```python
from build123d import *

# Parameters (mm, degrees)
PAD_DEPTH       = 30
POCKET_DEPTH    = 5
FILLET_R        = 14.5
FILLET001_R     = 14.5
FILLET002_R     = 12
SKETCH002_W     = 50.00223
SKETCH002_H     = 7.321129
PAD001_DEPTH    = 25
SKETCH003_R     = 4.8367523299
POCKET001_DEPTH = 10


with BuildPart() as part:
    # Sketch → Pad (new body)
    with BuildSketch(Plane.XY):
        Polygon((-26.0423896161, -2.4126467386), (-26.0423896161, 2.4126467386), (26.0423896161, 2.4126467386), (70.4083759206, -14.101078257), (69.0323338509, -17.9166155839), (26.0423896161, -2.4126467386), align=None)
    extrude(amount=PAD_DEPTH)

    # Sketch001 (on Face3 of Pad) → Pocket (cut)
    with BuildSketch(Plane(origin=(3.9577363848, 10.6329055553, 0), x_dir=(-0.9371842108, 0.3488348534, 0), z_dir=(0.3488348534, 0.9371842108, 0))):
        with BuildLine():
            ThreePointArc((-57.051074, 19.2972875988), (-61.3483615988, 15), (-57.051074, 10.7027124012))
            Line((-57.051074, 10.7027124012), (-38.086853, 10.7027124012))
            ThreePointArc((-38.086853, 10.7027124012), (-33.7895654012, 15), (-38.086853, 19.2972875988))
            Line((-38.086853, 19.2972875988), (-57.051074, 19.2972875988))
        make_face()
    extrude(amount=-POCKET_DEPTH, mode=Mode.SUBTRACT)

    # Fillet
    fillet_edges = [part.edges().sort_by_distance(p)[0] for p in [
        (69.720355, -16.008847, 30),
    ]]
    fillet(fillet_edges, radius=FILLET_R)

    # Fillet001
    fillet001_edges = [part.edges().sort_by_distance(p)[0] for p in [
        (69.720355, -16.008847, 0),
    ]]
    fillet(fillet001_edges, radius=FILLET001_R)

    # Fillet002
    fillet002_edges = [part.edges().sort_by_distance(p)[0] for p in [
        (26.04239, 2.412647, 15),
    ]]
    fillet(fillet002_edges, radius=FILLET002_R)

    # Sketch002 (on Face12 of Fillet002) → Pad001 (join)
    with BuildSketch(Plane(origin=(0, 2.4126467386, 0), x_dir=(-1, 0, 0), z_dir=(0, 1, 0))):
        with Locations((1.1177492, 26.194347)):
            Rectangle(SKETCH002_W, SKETCH002_H)
    extrude(amount=PAD001_DEPTH)

    # Sketch003 (on Face17 of Pad001) → Pocket001 (cut)
    with BuildSketch(Plane.XY.offset(29.8549115)):
        with Locations((10.379424, 18.289026)):
            Circle(SKETCH003_R)
        with BuildLine():
            Line((-30.0109383074, -0.5137681689), (-30.0109383074, 32.26572))
            Line((31.0117, 32.26572), (-30.0109383074, 32.26572))
            Line((32.17643, 11.966219), (31.0117, 32.26572))
            Line((23.690575, 12.964556), (32.17643, 11.966219))
            ThreePointArc((23.690575, 12.964556), (14.0178466447, 26.3039488372), (-2.2418022126, 23.6346991039))
            Line((-2.2418022126, 23.6346991039), (-30.0109383074, -0.5137681689))
        make_face()
    extrude(amount=-POCKET001_DEPTH, mode=Mode.SUBTRACT)


solid = part.part
```
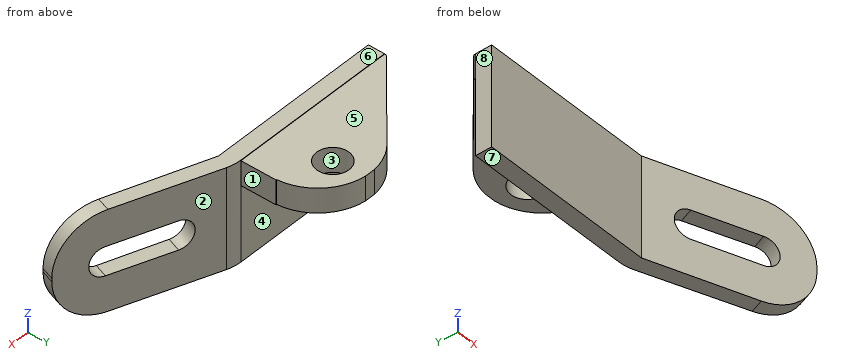
Here's how the part is built. I have some questions about the finished solid (model axes, mm). Face numbers are marked on the shaded views. A direction names the side the tool comes from. Coordinates: 2 decimals unless noted, no trailing zeros. Loops run counter-clockwise (first coordinate to the right, second up) from the corner with the lowest first, then second, coordinate; pieces in that order, holes last. Notation, with made-up numbers: (24.5, 4) - (66.5, 4) arc R25 cw to (66.5, 16) - close; hole circle Ø11 at (62, -25). An arc over 180 degrees is marked (long way). Return JSON: item names as keys, results as strings. Group by question number.
Item 1: If we section it at C-C on y = 17: Write out the boundary of the cut face in (x, z), and give its area (3 significant figures).
Item 2: If we section it at A-A on z = 24: Write out the boundary of the cut face in (x, y), and give its area (3 significant figures).
Item 3: Will these pins go through, and if not, where does the flat tip stop? P1, Ø15, axis at x = -7, z = 14, coming from the -Y side; P2, Ø2, axis at y = -3, z = 6, coming from the -X side; P3, Ø5, axis at x = 15.5, z = 21, coming from the +Y side.
Item 4: If we section it at B-B on x = 50.5: Write out the boundary of the cut face in (y, z).
Item 5: If we section it at D-D on x = -8: Write out the boundary of the cut face in (y, z), and give its area (3 significant figures).
Item 6: On a 3-axis mill with a long thin cutter (end or side, diameter ignored), from which of +Z, -Z, +X, -X, +Y, -Y can I reach the whole of each face in a straight line? I mean the marked faces 4, 5, 6, 7 and 8. Say none if no direction works.
Item 7: I need wall thicknesses on line 1 (Z direction, x = 3.5, y = 23); line 2 (Y direction, x = -5, z = 3.5); line 3 (Y direction, x = 66.5, z = 20). Which ranges of each line are inside material? Lowest first, please. Write a range as from..to.
Item 8: We'd pull the mould along Y, two halves only. Please class the marked faces 1, 2 and 3: +Y half, -Y half, draft (parallel to the pull), parting line (faces both ways), or undercut.
Calculated:
{
 "1": {"outline": "(-9.87, 22.53) - (5.72, 22.53) - (5.72, 29.85) - (-9.87, 29.85) - close; (15.04, 22.53) - (22.85, 22.53) - (22.85, 29.85) - (15.04, 29.85) - close", "area": "171 mm^2"},
 "2": {"outline": "(-26.12, 2.41) - (-26.04, 2.41) - (-26.04, -2.41) - (26.04, -2.41) - (66.44, -16.98) - (67.83, -13.14) - (28.07, 1.66) arc R12 ccw to (23.88, 2.41) - (23.88, 12.94) - (23.69, 12.96) arc R15.68 ccw to (9.54, 27.41) - (6.56, 27.41) arc R15.68 ccw to (-2.24, 23.63) - (-26.12, 2.87) - close; hole circle Ø9.67 at (10.38, 18.29)", "area": "1,210 mm^2"},
 "3": {"P1": "stops at y = -2.41", "P2": "stops at x = -26.04", "P3": "stops at y = 26.5"},
 "4": {"outline": "(-11.23, 0) - (-6.69, 0) - (-6.69, 10.7) - (-11.23, 10.7) - close; (-11.23, 19.3) - (-6.69, 19.3) - (-6.69, 30) - (-11.23, 30) - close"},
 "5": {"outline": "(-2.41, 0) - (2.41, 0) - (2.41, 22.53) - (18.63, 22.53) - (18.63, 29.85) - (2.41, 29.85) - (2.41, 30) - (-2.41, 30) - close", "area": "263 mm^2"},
 "6": {"face 4": "-Z, +X, -X, +Y", "face 5": "+Z, +X, -X, +Y", "face 6": "+Z, +X, -X, +Y, -Y", "face 7": "-Z, +X, -X, +Y, -Y", "face 8": "+Z, -Z, -X, -Y"},
 "7": {"line 1": "z = 22.53..29.85", "line 2": "y = -2.41..2.41", "line 3": "y = -17..-12.65"},
 "8": {"face 1": "draft", "face 2": "+Y half", "face 3": "undercut"}
}
